Could you check a few things on this model? Use its own coordinates, in mm. A direction names the side the tool comes from. Give positions to 0.01 mm unless a question says otherwise; leave off trailing zeros. Loops run counter-clockwise (first coordinate to the right, second up) from the corner with the lowest first, then second, coordinate; pieces in that order, holes last. Notation, with made-up numbers: M -8.5,69.25 L 2.5,69.25 A16 cw 2.5,81.25 Z; hole C 13,-26.5 d10. An arc over 180 degrees is marked long. Use CSV: the item, a comma, the result in double quotes.
```python
from build123d import *

# Parameters (mm, degrees)
F0_W          = 304.8
F0_H          = 25.4
F1_DEPTH      = 6.35
F2_R          = 12.69999
F3_R          = 4.7625
F4_DEPTH      = 12.701
F5_W          = 19.05
F5_H          = 6.35
F6_DEPTH      = 152.401
F6_DEPTH_BACK = 152.401


# Not quite as in the source:
# - a fillet or chamfer is up to 0.001 mm smaller than in the source, because OpenCascade refuses the exact size


with BuildPart() as f1:
    # F0 (on Top) → F1 (new body, symmetric)
    with BuildSketch(Plane.XY):
        Rectangle(F0_W, F0_H)
    extrude(amount=F1_DEPTH, both=True)

    # F2 (radius 12.7 in the source; OpenCascade refuses exactly that, so slightly less here)
    f2_edges = [f1.edges().sort_by_distance(p)[0] for p in [
        (-152.4, 12.7, 0),
        (-152.4, -12.7, 0),
        (152.4, 12.7, 0),
        (152.4, -12.7, 0),
    ]]
    fillet(f2_edges, radius=F2_R)

    # F3 (on face) → F4 (cut, through all)
    with BuildSketch(Plane.XY.offset(6.35)):
        with Locations((-139.7, 0)):
            Circle(F3_R)
        with Locations((139.7, 0)):
            Circle(F3_R)
    extrude(amount=-F4_DEPTH, mode=Mode.SUBTRACT)

    # F5 (on Right) → F6 (cut, two sides)
    with BuildSketch(Plane.YZ) as f6_sk:
        Rectangle(F5_W, F5_H)
    extrude(amount=-F6_DEPTH, mode=Mode.SUBTRACT)
    extrude(f6_sk.sketch, amount=F6_DEPTH_BACK, mode=Mode.SUBTRACT)


solid = f1.part
```
1. Which directions (+Z, -Z, +X, -X, +Y, -Y) give clear straight access to the entire face, cutting with the end or side of a thin tool? Please do faces 1 (the face through (134.942, 0.209, 4.785)), 2 (the face through (2, 9.525, 0)).
Outcome:
face 1,"+Z, -Z"
face 2,"+X, -X"
2. Please list where these lines run through material, in increasing order: line 1 (X direction, y = 0.75, z = -4.5); line 2 (Y direction, x = 83.5, z = 2.25) (3 decimals); line 3 (Y direction, x = -139.7, z = -4.7).
Outcome:
line 1,"-152.38 to -144.4, -135 to 135, 144.4 to 152.38"
line 2,"-12.7 to -9.525, 9.525 to 12.7"
line 3,"-12.7 to -4.76, 4.76 to 12.7"
3. I want a section at B-B, the plane x = -60. List the corners of the cut face in (y, z) for me (3 decimals).
Outcome:
outline,"M -12.7,-6.35 L 12.7,-6.35 L 12.7,6.35 L -12.7,6.35 Z; hole M -9.525,-3.175 L 9.525,-3.175 L 9.525,3.175 L -9.525,3.175 Z"
4. I want a section at A-A, the plane z = -0.5. List the corners of the cut face in (x, y) for me (3 decimals), then the cut area to 3 significant figures.
Outcome:
outline,"M -148.1,-9.525 A12.7 ccw -139.7,-12.7 L 139.7,-12.7 A12.7 ccw 148.1,-9.525 Z; M -148.1,9.525 L 148.1,9.525 A12.7 ccw 139.7,12.7 L -139.7,12.7 A12.7 ccw Z"
area,"1,850 mm2"
5. I'm going to push flat-ended pins straight in: pin 1 Ø7.5 at (x, y) = (-139.7, 0) entering from +Z; pin 2 Ø6 at (y, z) = (8.5, 0.5) entering from +X. Where does each tip first touch, or does it pass through?
Outcome:
pin 1,"through"
pin 2,"x = 150.2"
6. If we mould it in two halves opening along Y, with no side actions, what happens to faces 3 (the face through (2, 0, -3.175)), 4 (the face through (2, 0, 3.175)), 5 (the face through (-147.1, -10.32, 0.09)), 6 (the face through (147.1, 10.32, -0.09))? For each: +Y half, -Y half, draft (parallel to the pull), parting line (faces both ways), or undercut.
Outcome:
face 3,"undercut"
face 4,"undercut"
face 5,"-Y half"
face 6,"+Y half"
